```python
from build123d import *

# Parameters (mm, degrees)
F0_W     = 927.1
F0_H     = 127
F1_DEPTH = 19.05
F2_W     = 927.1
F2_H     = 19.05
F3_DEPTH = 6.35
F4_R     = 1.5875
F5_DEPTH = 19.051


with BuildPart() as f1:
    # F0 (on Front) → F1 (new body)
    with BuildSketch(Plane.XZ):
        with Locations((463.55, -63.5)):
            Rectangle(F0_W, F0_H)
    extrude(amount=F1_DEPTH)

    # F2 (on Front) → F3 (cut)
    with BuildSketch(Plane.XZ):
        with Locations((463.55, -111.125)):
            Rectangle(F2_W, F2_H)
    extrude(amount=F3_DEPTH, mode=Mode.SUBTRACT)

    # F4 (on Front) → F5 (cut, through all)
    with BuildSketch(Plane.XZ):
        with BuildLine():
            ThreePointArc((908.3203580187, -112.6893090461), (909.264361891, -112.1474878717), (909.6375, -111.125))
            ThreePointArc((909.6375, -111.125), (908.3283195264, -109.5620878172), (906.5600896174, -110.5769823892))
            ThreePointArc((906.5600896174, -110.5769823892), (907.8529355077, -110.9269295443), (908.417947636, -112.1412914353))
            ThreePointArc((908.417947636, -112.1412914353), (908.3933598189, -112.4196109618), (908.3203580187, -112.6893090461))
        make_face()
        with BuildLine():
            ThreePointArc((908.417947636, -112.1412914353), (907.8529355077, -110.9269295443), (906.5600896174, -110.5769823892))
            ThreePointArc((906.5600896174, -110.5769823892), (906.830447636, -112.1412914353), (908.3203580187, -112.6893090461))
            ThreePointArc((908.3203580187, -112.6893090461), (908.3933598189, -112.4196109618), (908.417947636, -112.1412914353))
        make_face()
        with BuildLine():
            ThreePointArc((908.3203580187, -112.6893090461), (906.830447636, -112.1412914353), (906.5600896174, -110.5769823892))
            ThreePointArc((906.5600896174, -110.5769823892), (905.6108952721, -113.1575828707), (908.3203580187, -112.6893090461))
        make_face()
        with Locations((730.25, -111.125)):
            Circle(F4_R)
        with Locations((552.45, -111.125)):
            Circle(F4_R)
        with Locations((374.65, -111.125)):
            Circle(F4_R)
        with Locations((196.85, -111.125)):
            Circle(F4_R)
        with Locations((19.05, -111.125)):
            Circle(F4_R)
    extrude(amount=F5_DEPTH, mode=Mode.SUBTRACT)


solid = f1.part
```
Work out the finished part from the listing and answer in its coordinate system (mm). Give positions to 0.01 mm unless a question says otherwise; leave off trailing zeros. Order: outer loops, then holes, each group sorted by start corner. A loop starts at its lowest first (then second) coordinate and runs counter-clockwise, first axis right, second up.
1. Section A-A, the plane x = 333.5 is taken. Determine the outline of the cut face in (y, z), and give its area (3 significant figures).
Result sheet:
outline: (-19.05, -127) - (0, -127) - (0, -120.65) - (-6.35, -120.65) - (-6.35, -101.6) - (0, -101.6) - (0, 0) - (-19.05, 0) - close
area: 2,300 mm2
2. Each of these flat-tipped pins is pushed along its axis until it touches: P1, Ø3, axis at x = 906.83, z = -112.14, coming from the -Y side; P2, Ø12, axis at x = 137.5, z = -62, coming from the +Y side; P3, Ø3, axis at x = 331.5, z = -113, coming from the +Y side. Where does it stop, or does it pass through?
Result sheet:
P1: passes through
P2: stops at y = 0
P3: stops at y = -6.35
3. Straight lines are drawn through the part: L1, parallel to Z at x = 387, y = -1.75; L2, parallel to Z at x = 374.65, y = -13.75; L3, parallel to Y at x = 492, z = -102. For each, find the intervals that lie inside material, in ascending order.
Result sheet:
L1: z = -127 to -120.65, -101.6 to 0
L2: z = -127 to -112.71, -109.54 to 0
L3: y = -19.05 to -6.35
4. The mould has two halves that part along Z. Classify faces 1 (the flat face through (457, -6.35, -111)), 2 (the flat face through (457, -9, 0)), 3 (the flat face through (0, -9, -64)): released by +Z, released by -Z, zero draft, split by the parting line, or undercut.
Result sheet:
face 1: undercut
face 2: released by +Z
face 3: zero draft
